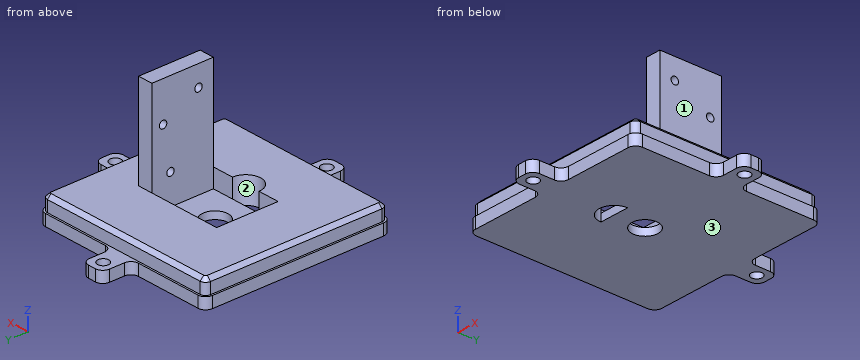
from build123d import *

# Parameters (mm, degrees)
SKETCH1_W           = 50
SKETCH1_H           = 50
BOSS_EXTRUDE1_DEPTH = 7
SKETCH3_W           = 19.5
SKETCH3_H           = 16.5
CUT_EXTRUDE1_DEPTH  = 5
SKETCH4_R           = 3.5
CUT_EXTRUDE2_DEPTH  = 5
CUT_EXTRUDE4_DEPTH  = 37.041642582
SKETCH6_W           = 4
SKETCH6_H           = 16.5
BOSS_EXTRUDE2_DEPTH = 25
SKETCH7_R           = 1
CUT_EXTRUDE5_DEPTH  = 57.129871726
SKETCH10_W          = 6
SKETCH10_H          = 8
SKETCH10_R          = 1.5
SKETCH10_W_2        = 8
SKETCH10_H_2        = 6
BOSS_EXTRUDE3_DEPTH = 3
FILLET1_R           = 2
FILLET2_R           = 2
CUT_EXTRUDE6_DEPTH  = 4
CHAMFER1_SIZE       = 1


with BuildPart() as part:
    # Sketch1 → Boss-Extrude1 (new body)
    with BuildSketch(Plane.XY):
        Rectangle(SKETCH1_W, SKETCH1_H)
    extrude(amount=BOSS_EXTRUDE1_DEPTH)

    # Sketch3 → Cut-Extrude1 (cut)
    with BuildSketch(Plane.XY.offset(7)):
        Rectangle(SKETCH3_W, SKETCH3_H)
    extrude(amount=-CUT_EXTRUDE1_DEPTH, mode=Mode.SUBTRACT)

    # Sketch4 → Cut-Extrude2 (cut)
    with BuildSketch(Plane.XY.offset(2)):
        Circle(SKETCH4_R)
    extrude(amount=-CUT_EXTRUDE2_DEPTH, mode=Mode.SUBTRACT)

    # Sketch5 → Cut-Extrude4 (cut, through all)
    with BuildSketch(Plane.XY.offset(7)):
        with BuildLine():
            Line((-4, -8.25), (4, -8.25))
            ThreePointArc((4, -8.25), (0, -12.25), (-4, -8.25))
        make_face()
    extrude(amount=-CUT_EXTRUDE4_DEPTH, mode=Mode.SUBTRACT)

    # Sketch6 → Boss-Extrude2 (add)
    with BuildSketch(Plane.XY.offset(7)):
        with Locations((11.75, 0)):
            Rectangle(SKETCH6_W, SKETCH6_H)
    extrude(amount=BOSS_EXTRUDE2_DEPTH)

    # Sketch7 → Cut-Extrude5 (cut, through all)
    with BuildSketch(Plane(origin=(13.75, 0, 0), x_dir=(0, 0, -1), z_dir=(1, 0, 0))):
        with Locations((-10, 3.25)):
            Circle(SKETCH7_R)
        with Locations((-26.5, -4.25)):
            Circle(SKETCH7_R)
        with Locations((-21.5, 5.25)):
            Circle(SKETCH7_R)
    extrude(amount=-CUT_EXTRUDE5_DEPTH, mode=Mode.SUBTRACT)

    # Sketch10 → Boss-Extrude3 (add)
    # profile 1 of 3: a face of its own
    with BuildSketch(Plane(origin=(0, 0, 0), x_dir=(-1, 0, 0), z_dir=(0, 0, -1))):
        with Locations((0, 29)):
            Rectangle(SKETCH10_W, SKETCH10_H)
        with Locations((0, 30)):
            Circle(SKETCH10_R, mode=Mode.SUBTRACT)
    # profile 2 of 3: a face of its own
    with BuildSketch(Plane(origin=(0, 0, 0), x_dir=(-1, 0, 0), z_dir=(0, 0, -1))):
        with Locations((-29, 0)):
            Rectangle(SKETCH10_W_2, SKETCH10_H_2)
        with Locations((-30, 0)):
            Circle(SKETCH10_R, mode=Mode.SUBTRACT)
    # profile 3 of 3: a face of its own
    with BuildSketch(Plane(origin=(0, 0, 0), x_dir=(-1, 0, 0), z_dir=(0, 0, -1))):
        with Locations((0, -29)):
            Rectangle(SKETCH10_W, SKETCH10_H)
        with Locations((0, -30)):
            Circle(SKETCH10_R, mode=Mode.SUBTRACT)
    extrude(amount=-BOSS_EXTRUDE3_DEPTH)

    # Fillet1
    fillet1_edges = [part.edges().sort_by_distance(p)[0] for p in [
        (3, -25, 1.5),
        (-3, -25, 1.5),
        (-3, -33, 1.5),
        (3, -33, 1.5),
        (25, 3, 1.5),
        (25, -3, 1.5),
        (33, -3, 1.5),
        (33, 3, 1.5),
        (-3, 25, 1.5),
        (3, 25, 1.5),
        (3, 33, 1.5),
        (-3, 33, 1.5),
    ]]
    fillet(fillet1_edges, radius=FILLET1_R)

    # Fillet2
    fillet2_edges = [part.edges().sort_by_distance(p)[0] for p in [
        (25, -25, 3.5),
        (-25, -25, 3.5),
        (-25, 25, 3.5),
        (25, 25, 3.5),
    ]]
    fillet(fillet2_edges, radius=FILLET2_R)

    # Sketch11 → Cut-Extrude6 (cut)
    with BuildSketch(Plane.XY.offset(7)):
        with BuildLine():
            Line((23, 25), (-23, 25))
            ThreePointArc((-23, 25), (-24.414213562, 24.414213562), (-25, 23))
            Line((-25, 23), (-25, -23))
            ThreePointArc((-25, -23), (-24.414213562, -24.414213562), (-23, -25))
            Line((-23, -25), (23, -25))
            ThreePointArc((23, -25), (24.414213562, -24.414213562), (25, -23))
            Line((25, -23), (25, 23))
            ThreePointArc((25, 23), (24.414213562, 24.414213562), (23, 25))
        make_face()
        with BuildLine():
            Line((23, 24.5), (-23, 24.5))
            ThreePointArc((-23, 24.5), (-24.060660172, 24.060660172), (-24.5, 23))
            Line((-24.5, 23), (-24.5, -23))
            ThreePointArc((-24.5, -23), (-24.060660172, -24.060660172), (-23, -24.5))
            Line((-23, -24.5), (23, -24.5))
            ThreePointArc((23, -24.5), (24.060660172, -24.060660172), (24.5, -23))
            Line((24.5, -23), (24.5, 23))
            ThreePointArc((24.5, 23), (24.060660172, 24.060660172), (23, 24.5))
        make_face(mode=Mode.SUBTRACT)
    extrude(amount=-CUT_EXTRUDE6_DEPTH, mode=Mode.SUBTRACT)

    # Chamfer1
    chamfer1_edges = [part.edges().sort_by_distance(p)[0] for p in [
        (0, 24.5, 7),
        (-24.060660172, 24.060660172, 7),
        (-24.5, 0, 7),
        (-24.060660172, -24.060660172, 7),
        (0, -24.5, 7),
        (24.060660172, -24.060660172, 7),
        (24.5, 0, 7),
        (24.060660172, 24.060660172, 7),
    ]]
    chamfer(chamfer1_edges, length=CHAMFER1_SIZE)


solid = part.part
Could you check a few things on this model? Use its own coordinates, in mm. Face numbers are marked on the shaded views. Coordinates: 2 decimals unless noted, no trailing zeros. Write each loop counter-clockwise with the first axis right and the second up, starting at its lowest first coordinate (ties: lowest second). Pieces come first, ordered by that corner, then holes. Notation, with made-up numbers: M -38.75,-18 L -7.75,-18 A28 cw -7.75,11 Z; hole C 55,6 d7. An arc over 180 degrees is marked long. One line per question, with ' | ' between items.
1) Imagine slicing it at C-C, the plane x = -15. Write out the boundary of the cut face in (y, z), and give its area (3 significant figures).
Checks:
outline: M -25,0 L 25,0 L 25,3 L 24.5,3 L 24.5,6 L 23.5,7 L -23.5,7 L -24.5,6 L -24.5,3 L -25,3 Z | area: 345 mm²
2) Imagine slicing it at A-A, the plane z = 21.5. Write out the boundary of the cut face in (x, y), and give its area (3 significant figures).
Checks:
outline: M 9.75,-8.25 L 13.75,-8.25 L 13.75,4.25 L 9.75,4.25 Z; M 9.75,6.25 L 13.75,6.25 L 13.75,8.25 L 9.75,8.25 Z | area: 58.0 mm²
3) Imagine slicing it at D-D, the plane x = 0. Write out the boundary of the cut face in (y, z), and give its area (4 significant figures).
Checks:
outline: M -33,0 L -31.5,0 L -31.5,3 L -33,3 Z; M -28.5,0 L -12.25,0 L -12.25,7 L -23.5,7 L -24.5,6 L -24.5,3 L -28.5,3 Z; M -8.25,0 L -3.5,0 L -3.5,2 L -8.25,2 Z; M 3.5,0 L 28.5,0 L 28.5,3 L 24.5,3 L 24.5,6 L 23.5,7 L 8.25,7 L 8.25,2 L 3.5,2 Z; M 31.5,0 L 33,0 L 33,3 L 31.5,3 Z | area: 250.5 mm²
4) I need wall thicknesses on probe 1 along Y at (x, z) = (12, 10); probe 2 along Z at (x, y) = (7.5, 18); probe 3 along Z at (x, y) = (-7, 0.5). Which ranges of each line are inside material? Lowest first, please. Write a range as [from, to].
Checks:
probe 1: [-8.25, 2.25], [4.25, 8.25] | probe 2: [0, 7] | probe 3: [0, 2]
5) Imagine slicing it at B-B, the plane y = 0. Write out the boundary of the cut face in (x, z).
Checks:
outline: M -25,0 L -3.5,0 L -3.5,2 L -9.75,2 L -9.75,7 L -23.5,7 L -24.5,6 L -24.5,3 L -25,3 Z; M 3.5,0 L 28.5,0 L 28.5,3 L 24.5,3 L 24.5,6 L 23.5,7 L 13.75,7 L 13.75,32 L 9.75,32 L 9.75,2 L 3.5,2 Z; M 31.5,0 L 33,0 L 33,3 L 31.5,3 Z
6) For pin 1 Ø2.5 at (y, z) = (29, 2) entering from -X; pin 2 Ø1.5 at (y, z) = (13, 1.5) entering from +X; pin 3 Ø1.5 at (x, z) = (1.5, 4) entering from +Y; pin 4 Ø1.6 at (y, z) = (3.25, 10) entering from +X, each with a flat end and sliding along its axis, tell me the tip position at first contact or that it passes through.
Checks:
pin 1: x = -3 | pin 2: x = 25 | pin 3: y = 24.5 | pin 4: through
7) If we mould it in two halves opening along X, with no side actions, what happens to the marked faces 1, 2 and 3? For each: released by +X, released by -X, zero draft, split by the parting line, or undercut.
Checks:
face 1: released by +X | face 2: undercut | face 3: zero draft
